Read the model definition and answer for the solid it produces. Units are mm, in the model's axes. Face numbers are marked on the shaded views. A direction names the side the tool comes from. Coordinates: 2 decimals unless noted, no trailing zeros. Loops run counter-clockwise (first coordinate to the right, second up) from the corner with the lowest first, then second, coordinate; pieces in that order, holes last. Notation, with made-up numbers: (-39.75, 80) -> (-3.75, 80) arc R33 ccw to (-3.75, 118) -> close; hole circle Ø7 at (57.25, -4.75). An arc over 180 degrees is marked (long way). Answer as a JSON object with one key per item and string values. Group by question number.
Q1. Straight lines are drawn through the part: line 1 along X through (y, z) = (1.35, -5.25); line 2 along Z through (x, y) = (6, 31); line 3 along Y through (x, z) = (11.25, -5.5). For each, find the intervals that lie inside material, in ascending order. Write a range as [from, to].
Q2. Each of these flat-tipped pins is pushed along its axis until it touches: P1, Ø4, axis at x = 8.5, y = 17, coming from the +Z side; P2, Ø2.5, axis at x = 7, z = -5.25, coming from the +Y side; P3, Ø1.5, axis at x = 3, z = -1.5, coming from the -Y side; P4, Ø3, axis at x = 3, z = -5, coming from the +Y side. Where does it stop, or does it pass through?
Q3. For the marked faces 1 and 2, determine the directions among +Z, -Z, +X, -X, +Y, -Y from which every point of the face is accessible in a straight line to the end or side of a thin tool.
Q4. The part is cut by section B-B on x = 7. Write down the section's boundary in (y, z), and give its area (3 significant figures).
Q5. The part is cut by section D-D on y = 24. Write down the section's boundary in (x, z), and give its area (3 significant figures).
Q6. The part is cut by section A-A on z = -5.25. Write down the section's boundary in (x, y).
Q7. The part is cut by section C-C on x = 20.25. Write down the section's boundary in (y, z), and give its area (3 significant figures).
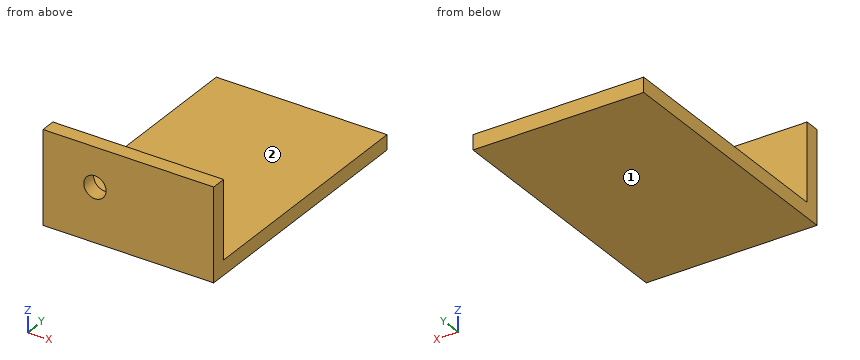
from build123d import *

# Parameters (mm, degrees)
SKETCH1_W           = 23
SKETCH1_H           = 12.5
BOSS_EXTRUDE1_DEPTH = 2
SKETCH2_W           = 23
SKETCH2_H           = 33.206230298
BOSS_EXTRUDE2_DEPTH = 2
SKETCH3_R           = 1.5
CUT_EXTRUDE1_DEPTH  = 2


with BuildPart() as part:
    # Sketch1 → Boss-Extrude1 (new body)
    with BuildSketch(Plane(origin=(0, 0, 0), x_dir=(1, 0, 0), z_dir=(0, 1, 0))):
        with Locations((11.5, 6.25)):
            Rectangle(SKETCH1_W, SKETCH1_H)
    extrude(amount=BOSS_EXTRUDE1_DEPTH)

    # Sketch2 → Boss-Extrude2 (add)
    with BuildSketch(Plane(origin=(0, 0, -12.5), x_dir=(-1, 0, 0), z_dir=(0, 0, -1))):
        with Locations((-11.5, 18.603115149)):
            Rectangle(SKETCH2_W, SKETCH2_H)
    extrude(amount=-BOSS_EXTRUDE2_DEPTH)

    # Sketch3 → Cut-Extrude1 (cut)
    with BuildSketch(Plane(origin=(0, 2, 0), x_dir=(1, 0, 0), z_dir=(0, 1, 0))):
        with Locations(Location((7, 5.25, 0), (0, 0, 270))):
            Circle(SKETCH3_R)
    extrude(amount=-CUT_EXTRUDE1_DEPTH, mode=Mode.SUBTRACT)


solid = part.part
Final values:
{
 "1": {"line 1": "x = [0, 5.5], [8.5, 23]", "line 2": "z = [-12.5, -10.5]", "line 3": "y = [0, 2]"},
 "2": {"P1": "stops at z = -10.5", "P2": "passes through", "P3": "stops at y = 0", "P4": "stops at y = 2"},
 "3": {"face 1": "-Z, +X, -X, +Y, -Y", "face 2": "+Z, +X, -X, +Y"},
 "4": {"outline": "(0, -12.5) -> (35.21, -12.5) -> (35.21, -10.5) -> (2, -10.5) -> (2, -6.75) -> (0, -6.75) -> close; (0, -3.75) -> (2, -3.75) -> (2, 0) -> (0, 0) -> close", "area": "85.4 mm2"},
 "5": {"outline": "(0, -12.5) -> (23, -12.5) -> (23, -10.5) -> (0, -10.5) -> close", "area": "46.0 mm2"},
 "6": {"outline": "(0, 0) -> (5.5, 0) -> (5.5, 2) -> (0, 2) -> close; (8.5, 0) -> (23, 0) -> (23, 2) -> (8.5, 2) -> close"},
 "7": {"outline": "(0, -12.5) -> (35.21, -12.5) -> (35.21, -10.5) -> (2, -10.5) -> (2, 0) -> (0, 0) -> close", "area": "91.4 mm2"}
}
